```python
from build123d import *

# Parameters (mm, degrees)
BOSS_EXTRU_1_DEPTH = 15
TROU_TARAUD_M101_D = 8.5
CONG_1_R           = 10


with BuildPart() as part:
    # Esquisse1 → Boss.-Extru.1 (new body)
    with BuildSketch(Plane.XY):
        with BuildLine():
            Line((0, 0), (0, 60))
            Line((0, 60), (30, 60))
            Line((30, 60), (30, 0))
            ThreePointArc((30, 0), (15, 6.771243445), (0, 0))
        make_face()
    extrude(amount=BOSS_EXTRU_1_DEPTH)

    # Trou taraudé M101 (through all)
    with Locations(Plane.XY.offset(15)):
        with Locations((15, 50)):
            Hole(TROU_TARAUD_M101_D / 2)

    # Congé1
    cong_1_edges = [part.edges().sort_by_distance(p)[0] for p in [
        (0, 60, 7.5),
        (30, 60, 7.5),
    ]]
    fillet(cong_1_edges, radius=CONG_1_R)


solid = part.part
```
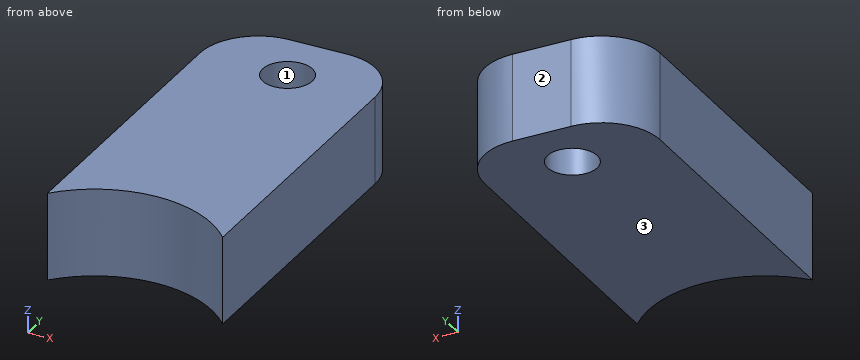
Can you work these out from the model? Positions are in its coordinate system, mm. Face numbers are marked on the shaded views. Coordinates: 2 decimals unless noted, no trailing zeros. Loops run counter-clockwise (first coordinate to the right, second up) from the corner with the lowest first, then second, coordinate; pieces in that order, holes last. Notation, with made-up numbers: M 60.5,52.5 L 95.5,52.5 A13 ccw 95.5,56.5 Z; hole C -40,-26.75 d9. An arc over 180 degrees is marked long. Put each result on its own line as item: value. Start each with the question number.
(1) Imagine slicing it at C-C on y = 5. List the corners of the cut face in (x, z) for me, and give its area (3 significant figures).
(2) We'd pull the mould along Y, two halves only. Please class the marked faces 1, 2 and 3: +Y half, -Y half, draft (parallel to the pull), parting line (faces both ways), or undercut.
(3) I need wall thicknesses on probe 1 along Y at (x, z) = (15, 9.5); probe 2 along Y at (x, z) = (18, 5.75); probe 3 along X at (y, z) = (3, 6.5). Which ranges of each line are inside material? Lowest first, please.
(4) Imagine slicing it at A-A on z = 9.25. List the corners of the cut face in (x, y) for me.
(5) Imagine slicing it at B-B on x = 17. List the corners of the cut face in (y, z) for me.
(6) Imagine slicing it at D-D on x = 23. List the corners of the cut face in (y, z) for me, and give its area (3 significant figures).
(7) Will these pins go through, and if not, where does the flat tip stop? pin 1 Ø5 at (x, y) = (7.5, 7.5) entering from -Z; pin 2 Ø7.5 at (x, y) = (15, 50) entering from -Z; pin 3 Ø2 at (x, z) = (14, 9.5) entering from -Y.
Worked answers:
1. outline: M 0,0 L 6.77,0 L 6.77,15 L 0,15 Z; M 23.23,0 L 30,0 L 30,15 L 23.23,15 Z
1. area: 203 mm2
2. face 1: undercut
2. face 2: +Y half
2. face 3: draft
3. probe 1: y = 6.77 to 45.75, 54.25 to 60
3. probe 2: y = 6.54 to 46.99, 53.01 to 60
3. probe 3: x = 0 to 3.31, 26.69 to 30
4. outline: M 0,0 A20 cw 30,0 L 30,50 A10 ccw 20,60 L 10,60 A10 ccw 0,50 Z; hole C 15,50 d8.5
5. outline: M 6.67,0 L 46.25,0 L 46.25,15 L 6.67,15 Z; M 53.75,0 L 60,0 L 60,15 L 53.75,15 Z
6. outline: M 5.1,0 L 59.54,0 L 59.54,15 L 5.1,15 Z
6. area: 817 mm2
7. pin 1: stops at z = 0
7. pin 2: passes through
7. pin 3: stops at y = 6.67
